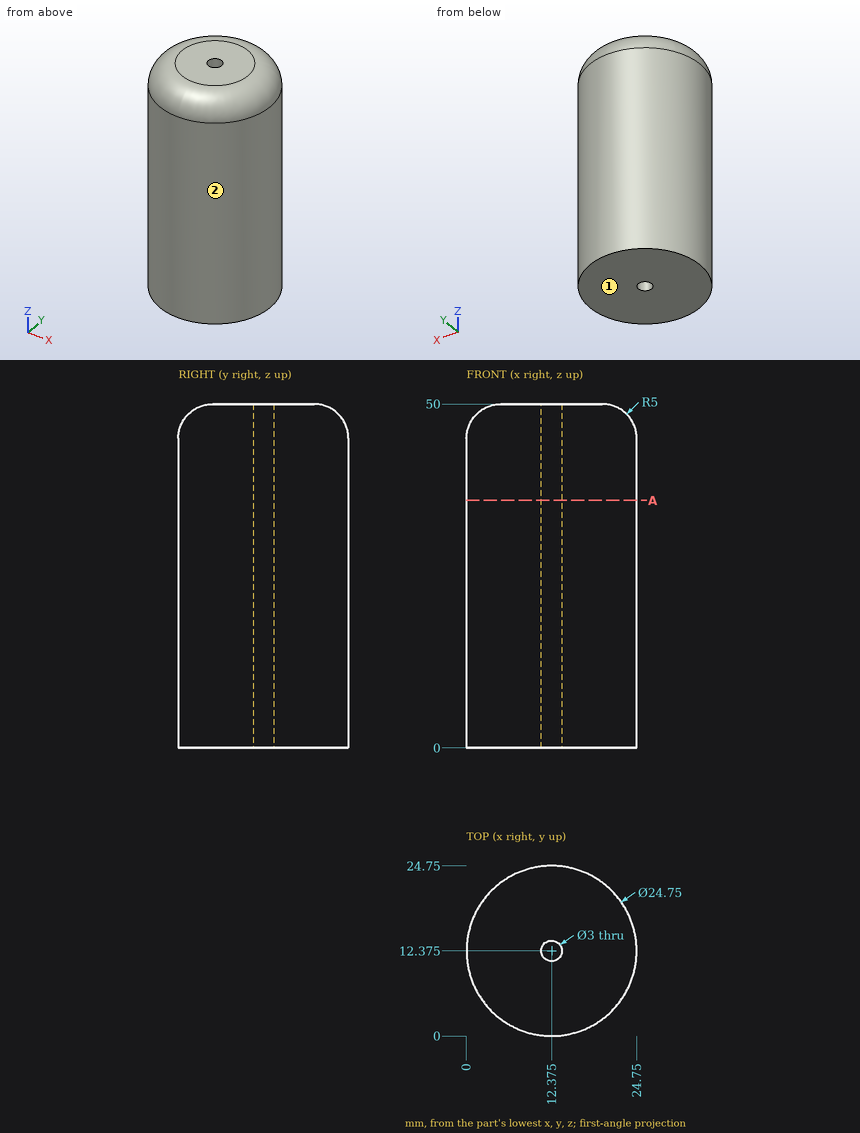
For this review, use the dimensioned drawing (mm, ordinates from the lowest corner) and the shaded views. Give positions to 0.01 mm unless a question says otherwise; leave off trailing zeros. Write each loop counter-clockwise with the first axis right and the second up, starting at its lowest first coordinate (ties: lowest second). Pieces come first, ordered by that corner, then holes. Notation, with made-up numbers: M -28.75,84.25 L -22.75,84.25 A13 cw -22.75,105.25 Z; hole C 68,-18 d3. An arc over 180 degrees is marked long. Answer as a JSON object with one key per item and string values. Group by question number.
1) Clearance check with flat-ended pins moving along their axes: pin 1 Ø10 at (y, z) = (21, 35) entering from -X; pin 2 Ø12 at (y, z) = (6, 14) entering from -X; pin 3 Ø12 at (y, z) = (3.5, 40) entering from -X; pin 4 Ø2.5 at (x, y) = (12.375, 12.375) entering from +Z. State where each tip first meets the part, or that it passes through.
2) We need section A-A (z = 36). Give the boundary of the cut face in (x, y) (3 decimals).
3) Mouldability with a two-part tool opening along Y and no side actions: class the marked faces 1 and 2 as released by +Y, released by -Y, zero draft, split by the parting line, or undercut.
4) For line 1 along Y through (x, z) = (12.25, 8); line 2 along X through (y, z) = (19.25, 46); line 3 along X through (y, z) = (23.5, 43), list the stretches that pass through material, from the lowest coordinate up.
Answer key:
{
 "1": {"pin 1": "stops at x = 0.54", "pin 2": "stops at x = 0.01", "pin 3": "stops at x = 0.34", "pin 4": "passes through"},
 "2": {"outline": "C 12.375,12.375 d24.75; hole C 12.375,12.375 d3"},
 "3": {"face 1": "zero draft", "face 2": "split by the parting line"},
 "4": {"line 1": "y = 0 to 10.88, 13.87 to 24.75", "line 2": "x = 2.21 to 22.54", "line 3": "x = 6.96 to 17.79"}
}
